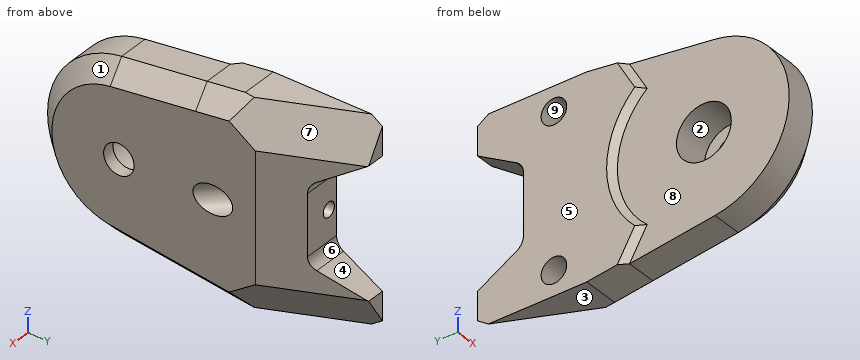
from build123d import *

# Parameters (mm, degrees)
BOSS_EXTRUDE4_DEPTH  = 4.5
SKETCH1_R            = 2.25
BOSS_EXTRUDE1_DEPTH  = 4
SKETCH1_4_R          = 2.25
SKETCH1_4_R_2        = 1.25
BOSS_EXTRUDE2_DEPTH  = 1
CHAMFER1_SIZE        = 3
CHAMFER1_SIZE_2      = 5.196152423
FILLET1_R            = 1.15
CHAMFER2_SIZE        = 7
CHAMFER2_SIZE2       = 3
CHAMFER3_SIZE        = 3
CHAMFER3_SIZE2       = 1.732050808
CHAMFER4_SIZE        = 1.5
CUT_EXTRUDE1_START   = -2
SKETCH1_6_R          = 1.05
CUT_EXTRUDE1_DEPTH   = 19.48660355
CUT_SWEEP1_PROFILE_R = 0.6
CUT_SWEEP2_PROFILE_R = 1.15
CHAMFER5_SIZE        = 0.5


# Some blends are built 0.0001 mm under size
with BuildPart() as part:
    # Sketch1<7> → Boss-Extrude4 (new body)
    with BuildSketch(Plane(origin=(0, 0, 0), x_dir=(0, 0, -1), z_dir=(1, 0, 0))):
        with BuildLine():
            Line((8.27, 9.234757272), (8.27, 18.195))
            Line((8.27, 18.195), (2.325, 18.195))
            Line((2.325, 18.195), (2.325, 14.425))
            Line((2.325, 14.425), (-2.325, 14.425))
            Line((-2.325, 14.425), (-2.325, 18.195))
            Line((-2.325, 18.195), (-8.27, 18.195))
            Line((-8.27, 18.195), (-8.27, 9.234757272))
            Line((-8.27, 9.234757272), (-7.859471067, 6.101983066))
            Line((-7.859471067, 6.101983066), (-5.358442733, 4.658013684))
            ThreePointArc((-5.358442733, 4.658013684), (0, 7.1), (5.358442733, 4.658013684))
            Line((5.358442733, 4.658013684), (7.859471067, 6.101983066))
            Line((7.859471067, 6.101983066), (8.27, 9.234757272))
        make_face()
    extrude(amount=-BOSS_EXTRUDE4_DEPTH)

    # Sketch1 → Boss-Extrude1 (add)
    with BuildSketch(Plane(origin=(0, 0, 0), x_dir=(0, 0, -1), z_dir=(1, 0, 0))):
        with BuildLine():
            Line((6.940659998, -0.909526687), (7.859471067, 6.101983066))
            Line((7.859471067, 6.101983066), (5.358442733, 4.658013684))
            ThreePointArc((5.358442733, 4.658013684), (0, 7.1), (-5.358442733, 4.658013684))
            Line((-5.358442733, 4.658013684), (-7.859471067, 6.101983066))
            Line((-7.859471067, 6.101983066), (-6.940659998, -0.909526687))
            ThreePointArc((-6.940659998, -0.909526687), (0, -7), (6.940659998, -0.909526687))
        make_face()
        Circle(SKETCH1_R, mode=Mode.SUBTRACT)
    extrude(amount=-BOSS_EXTRUDE1_DEPTH)

    # Sketch1<4> → Boss-Extrude2 (add)
    with BuildSketch(Plane(origin=(0, 0, 0), x_dir=(0, 0, -1), z_dir=(1, 0, 0))):
        Circle(SKETCH1_4_R)
        Circle(SKETCH1_4_R_2, mode=Mode.SUBTRACT)
    extrude(amount=-BOSS_EXTRUDE2_DEPTH)

    # Chamfer1
    # the kernel refuses this chamfer: 5.196152423, 3 mm, written as the material it takes off along each edge
    with BuildSketch(Plane(origin=(13.442891912, 18.195, -2.325), x_dir=(0, 0.057893862402672046, -0.9983227437537926), z_dir=(-1, 0, 0))) as chamfer1_piece_1_section:
        Polygon((CHAMFER1_SIZE * 0.998322743754, CHAMFER1_SIZE * 0.0578938624027), (-CHAMFER1_SIZE_2 * 0.0578938623994, CHAMFER1_SIZE_2 * 0.998322743697), (0, 0), align=None)
    chamfer1_piece_1 = extrude(amount=31.385783824, mode=Mode.PRIVATE)
    chamfer1_piece_1 = split(chamfer1_piece_1, bisect_by=Plane(origin=(-2.25, 14.425, -3.37149022), z_dir=(0, 1, 0)), keep=Keep.TOP, mode=Mode.PRIVATE)
    add(chamfer1_piece_1, mode=Mode.SUBTRACT)
    with BuildSketch(Plane(origin=(13.442891912, 18.195, 2.325), x_dir=(0, -0.9998132206222079, -0.019326765612700594), z_dir=(-1, 0, 0))) as chamfer1_piece_2_section:
        Polygon((CHAMFER1_SIZE_2 * 0.999813220566, CHAMFER1_SIZE_2 * 0.0193267656116), (-CHAMFER1_SIZE * 0.0193267656127, CHAMFER1_SIZE * 0.999813220622), (0, 0), align=None)
    chamfer1_piece_2 = extrude(amount=31.385783824, mode=Mode.PRIVATE)
    chamfer1_piece_2 = split(chamfer1_piece_2, bisect_by=Plane(origin=(-2.25, 14.425, 3.37149022), z_dir=(0, 1, 0)), keep=Keep.TOP, mode=Mode.PRIVATE)
    add(chamfer1_piece_2, mode=Mode.SUBTRACT)

    # Fillet1
    fillet1_edges = [part.edges().sort_by_distance(p)[0] for p in [
        (-2.25, 14.425, -3.148389485),
        (-2.25, 14.425, 3.148389485),
    ]]
    fillet(fillet1_edges, radius=FILLET1_R)

    # Chamfer2
    chamfer2_edges = [part.edges().sort_by_distance(p)[0] for p in [
        (0, 18.195, 6.7975),
    ]]
    chamfer2_side = [part.faces().sort_by_distance(p)[0] for p in [
        (0, 5.909970068, 0),
    ]]
    chamfer(chamfer2_edges, length=CHAMFER2_SIZE, length2=CHAMFER2_SIZE2, reference=chamfer2_side[0])

    # Chamfer3
    chamfer3_edges = [part.edges().sort_by_distance(p)[0] for p in [
        (-1.5, 14.695, -8.27),
        (-1.5, 14.695, 8.27),
    ]]
    chamfer3_side = [part.faces().sort_by_distance(p)[0] for p in [
        (-1.210290333, 14.019010778, 0),
    ]]
    chamfer(chamfer3_edges, length=CHAMFER3_SIZE, length2=CHAMFER3_SIZE2, reference=chamfer3_side[0])

    # Chamfer4
    chamfer4_edges = [part.edges().sort_by_distance(p)[0] for p in [
        (0, 3.140553901, 7.471395746),
        (0, 3.140553901, -7.471395746),
        (0, -7, 0),
    ]]
    chamfer(chamfer4_edges, length=CHAMFER4_SIZE)

    # Sketch1<6> → Cut-Extrude1 (cut, through all)
    with BuildSketch(Plane(origin=(0, 0, 0), x_dir=(0, 0, -1), z_dir=(1, 0, 0)).offset(CUT_EXTRUDE1_START)):
        with Locations((6.25, 11.925)):
            Circle(SKETCH1_6_R)
        with Locations((-6.25, 11.925)):
            Circle(SKETCH1_6_R)
    extrude(amount=-CUT_EXTRUDE1_DEPTH, mode=Mode.SUBTRACT)

    # Cut-Sweep1: sweep along a path in Sketch2
    with BuildLine(Plane.XY) as cut_sweep1_path:
        Line((4.128300859, 3.586165235), (-2.942766953, 10.657233047))
        ThreePointArc((-2.942766953, 10.657233047), (-3.484698831, 11.468291419), (-3.675, 12.425))
        Line((-3.675, 12.425), (-3.675, 14.425))
    # Cut-Sweep1 profile (on start of the path) → Cut-Sweep1 (sweep, cut)
    with BuildSketch(Plane(origin=(4.128300859, 3.586165235, 0), x_dir=(-0.7071067811865461, -0.707106781186549, 0), z_dir=(-0.707106781186549, 0.7071067811865461, 0))):
        Circle(CUT_SWEEP1_PROFILE_R)
    sweep(path=cut_sweep1_path.line, mode=Mode.SUBTRACT)

    # Cut-Sweep2: sweep along a path in Sketch2<3>
    with BuildLine(Plane.XY) as cut_sweep2_path:
        Line((-2.942766953, 10.657233047), (4.128300859, 3.586165235))
    # Cut-Sweep2 profile (on start of the path) → Cut-Sweep2 (sweep, cut)
    with BuildSketch(Plane(origin=(-2.942766953, 10.657233047, 0), x_dir=(0.7071067811865461, 0.707106781186549, 0), z_dir=(0.707106781186549, -0.7071067811865461, 0))):
        Circle(CUT_SWEEP2_PROFILE_R)
    sweep(path=cut_sweep2_path.line, mode=Mode.SUBTRACT)

    # Chamfer5
    chamfer5_edges = [part.edges().sort_by_distance(p)[0] for p in [
        (-4.5, 5.379998375, -6.6089569),
        (-4.5, 7.1, 0),
        (-4.5, 5.379998375, 6.6089569),
    ]]
    chamfer(chamfer5_edges, length=CHAMFER5_SIZE - 0.0001)  # a hair under: the kernel refuses the full size


solid = part.part
The listing builds one solid part. Answer for the finished solid, in the listing's coordinates (mm). Face numbers are marked on the shaded views. A direction names the side the tool comes from. Coordinates: 2 decimals unless noted, no trailing zeros. Loops run counter-clockwise (first coordinate to the right, second up) from the corner with the lowest first, then second, coordinate; pieces in that order, holes last. Notation, with made-up numbers: (57, -18.5) -> (110, -18.5) arc R22 ccw to (110, 13.5) -> close; hole circle Ø3 at (-3.75, 26). An arc over 180 degrees is marked (long way). Write item = value, one per line. Start each with the question number.
1) A cutting plane is placed at A-A (y = 16.25). Give the vertices of the cut face in (x, z), then the cut area to 3 significant figures.
2) A cutting plane is placed at D-D (y = 0). Give the vertices of the cut face in (x, z), then the cut area to 3 significant figures.
3) Straight lines are drawn through the part: line 1 (Z direction, x = -2.7, y = 12.5); line 2 (X direction, y = -1, z = -4.75); line 3 (Z direction, x = -2.8, y = 11). For each, find the intervals that lie inside material, in ascending order. Write a range as from..to.
4) Given pin 1 Ø4 at (y, z) = (0, 0) entering from +X; pin 2 Ø2 at (x, z) = (-2, 4) entering from -Y; pin 3 Ø0.9 at (x, z) = (-2.5, 0) entering from +Y (3 decimals); pin 4 Ø1.7 at (y, z) = (11.925, -6.25) entering from +X, each flat-ended and moving along its own axis, determine where each tip first touches the part or whether it passes through.
5) The mould has two halves that part along Y. Classify the marked faces 1, 2, 3 and 4: released by +Y, released by -Y, zero draft, split by the parting line, or undercut.
6) A cutting plane is placed at B-B (z = 0). Count the separate pieces of the cut face and the enclosed holes in it, then the cut area to 3 significant figures.
7) A tool of negligible diameter and unlimited length cuts with its end or side. For the marked faces 5, 6, 7, 8 and 9, from which of +Z, -Z, +X, -X, +Y, -Y can it reach the whole face along a straight path? Write none if from no direction.
Responses:
q1.outline = (-4.5, -8.27) -> (-4.05, -8.27) -> (-2.17, -5.27) -> (-2.17, -4.2) -> (-4.5, -4.2) -> close; (-4.5, 4.2) -> (-2.17, 4.2) -> (-2.17, 5.27) -> (-4.05, 8.27) -> (-4.5, 8.27) -> close
q1.area = 13.3 mm²
q2.outline = (-4, -7.06) -> (-1.5, -7.06) -> (0, -5.55) -> (0, -1.25) -> (-1, -1.25) -> (-1, -2.25) -> (-4, -2.25) -> close; (-4, 2.25) -> (-1, 2.25) -> (-1, 1.25) -> (0, 1.25) -> (0, 5.55) -> (-1.5, 7.06) -> (-4, 7.06) -> close
q2.area = 38.2 mm²
q3.line_1 = -8.27..-7.13, -5.37..5.37, 7.13..8.27
q3.line_2 = -4..0
q3.line_3 = -8.27..-6.75, -5.75..-0.5, 0.5..5.75, 6.75..8.27
q4.pin_1 = 0
q4.pin_2 = -6.32
q4.pin_3 = 14.425
q4.pin_4 = -0.28
q5.face_1 = released by -Y
q5.face_2 = undercut
q5.face_3 = zero draft
q5.face_4 = released by +Y
q6.separate_pieces = 3
q6.enclosed_holes = 0
q6.area = 55.5 mm²
q7.face_5 = +Z, -Z, -X, +Y, -Y
q7.face_6 = +X, -X, +Y
q7.face_7 = +Z, +X, +Y
q7.face_8 = -X, -Y
q7.face_9 = -X
